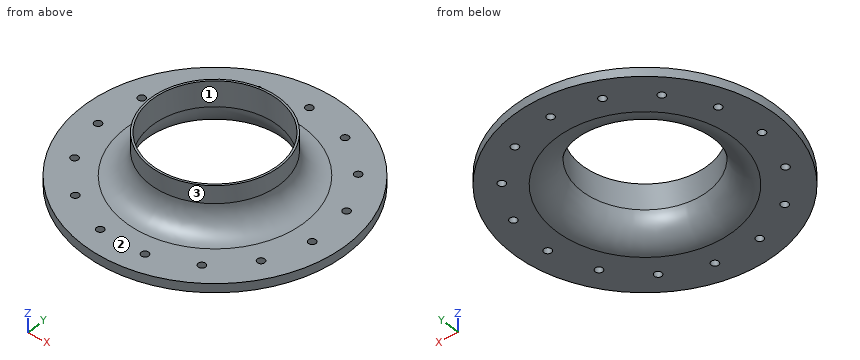
from build123d import *

# Parameters (mm, degrees)
ESQUISSE2_R             = 1.5
ENL_V_MAT_EXTRU_1_DEPTH = 78.521900132


with BuildPart() as part:
    # Esquisse1 → Base-Révolution (revolve)
    with BuildSketch(Plane(origin=(0, 0, 0), x_dir=(0, 0, -1), z_dir=(1, 0, 0)), mode=Mode.PRIVATE) as base_r_volution_sk:
        with BuildLine():
            Line((20.85, 46.5), (20.85, 53.45))
            Line((20.85, 53.45), (17.2, 53.45))
            Line((17.2, 53.45), (17.2, 36.3))
            ThreePointArc((17.2, 36.3), (14.271067812, 29.228932188), (7.2, 26.3))
            Line((7.2, 26.3), (0, 26.3))
            Line((0, 26.3), (0, 25.5))
            Line((0, 25.5), (1.5, 25.5))
            Line((1.5, 25.5), (10.35, 25.5))
            ThreePointArc((10.35, 25.5), (17.774621202, 28.575378798), (20.85, 36))
            Line((20.85, 36), (20.85, 46.5))
        make_face()
    revolve(base_r_volution_sk.sketch.rotate(Axis((0, 0, 0), (0, 0, -1)), 90), axis=Axis((0, 0, 0), (0, 0, -1)))

    # Esquisse2 → Enlèv. mat.-Extru.1 (cut, through all)
    with BuildSketch(Plane.XY.offset(-17.2)):
        with Locations((0, 44.5)):
            Circle(ESQUISSE2_R)
        with Locations((18.099780617, 40.652772865)):
            Circle(ESQUISSE2_R)
        with Locations((33.069944734, 29.776311983)):
            Circle(ESQUISSE2_R)
        with Locations((42.322014975, 13.75125625)):
            Circle(ESQUISSE2_R)
        with Locations((44.256224344, -4.651516615)):
            Circle(ESQUISSE2_R)
        with Locations((38.538130468, -22.25)):
            Circle(ESQUISSE2_R)
        with Locations((26.156443727, -36.00125625)):
            Circle(ESQUISSE2_R)
        with Locations((9.252070241, -43.527568233)):
            Circle(ESQUISSE2_R)
        with Locations((-9.252070241, -43.527568233)):
            Circle(ESQUISSE2_R)
        with Locations((-26.156443727, -36.00125625)):
            Circle(ESQUISSE2_R)
        with Locations((-38.538130468, -22.25)):
            Circle(ESQUISSE2_R)
        with Locations((-44.256224344, -4.651516615)):
            Circle(ESQUISSE2_R)
        with Locations((-42.322014975, 13.75125625)):
            Circle(ESQUISSE2_R)
        with Locations((-33.069944734, 29.776311983)):
            Circle(ESQUISSE2_R)
        with Locations((-18.099780617, 40.652772865)):
            Circle(ESQUISSE2_R)
    extrude(amount=-ENL_V_MAT_EXTRU_1_DEPTH, mode=Mode.SUBTRACT)


solid = part.part
Source: CAD feature listing. Evaluate the final solid. Frame: model axes, mm. Face numbers are marked on the shaded views. Round coordinates to 2 decimals unless told otherwise and drop trailing zeros. Loops run counter-clockwise (first coordinate to the right, second up) from the corner with the lowest first, then second, coordinate; pieces in that order, holes last. Notation, with made-up numbers: M 54,73.25 L 65,73.25 A16 ccw 65,84.25 Z; hole C 6.25,-26 d1. An arc over 180 degrees is marked long. Return JSON: item names as keys, results as strings. Group by question number.
1. Section query D-D on y = 44.5. Output: boundary loops of the cut face in (x, z), and give its area (3 significant figures).
2. Pin query (flat end, axial travel): pin 1 (12 mm diameter, centred on x = -18, z = -9, fed in from -Y); pin 2 (4 mm diameter, centred on x = 1.5, z = -3.5, fed in from -Y); pin 3 (5 mm diameter, centred on x = 2.5, z = -8, fed in from -Y). Return the tip coordinate at first contact, or that it passes through.
3. Section query C-C on z = -1.5. Output: boundary loops of the cut face in (x, y), and give its area (3 significant figures).
4. Section query A-A on x = 0. Output: boundary loops of the cut face in (y, z).
5. Material intervals for line 1 along Y through (x, z) = (-6.5, -4.5); line 2 along X through (y, z) = (15, -18.75); line 3 along X through (y, z) = (-12, -18.75), sorted ascending. Write a range as from..to.
6. Mould query, pull axis X, two halves, no side actions, for the marked faces 1, 2 and 3. Classes: released by +X, released by -X, zero draft, split by the parting line, or undercut.
7. Section query B-B on y = 0. Output: boundary loops of the cut face in (x, z), and give its area (3 significant figures).
Checks:
{
 "1": {"outline": "M -29.61,-20.85 L -1.5,-20.85 L -1.5,-17.2 L -29.61,-17.2 Z; M 1.5,-20.85 L 29.61,-20.85 L 29.61,-17.2 L 1.5,-17.2 Z", "area": "205 mm²"},
 "2": {"pin 1": "stops at y = -25.01", "pin 2": "stops at y = -26.3", "pin 3": "stops at y = -26.77"},
 "3": {"outline": "C 0,0 d52.6; hole C 0,0 d51", "area": "130 mm²"},
 "4": {"outline": "M -53.45,-20.85 L -36,-20.85 A10.5 ccw -25.5,-10.35 L -25.5,0 L -26.3,0 L -26.3,-7.2 A10 cw -36.3,-17.2 L -53.45,-17.2 Z; M 25.5,-10.35 A10.5 ccw 36,-20.85 L 43,-20.85 L 43,-17.2 L 36.3,-17.2 A10 cw 26.3,-7.2 L 26.3,0 L 25.5,0 Z; M 46,-20.85 L 53.45,-20.85 L 53.45,-17.2 L 46,-17.2 Z"},
 "5": {"line 1": "y = -25.48..-24.66, 24.66..25.48", "line 2": "x = -51.3..-43.15, -41.49..-25.63, 25.63..41.49, 43.15..51.3", "line 3": "x = -52.09..-27.17, 27.17..52.09"},
 "6": {"face 1": "undercut", "face 2": "zero draft", "face 3": "split by the parting line"},
 "7": {"outline": "M -53.45,-20.85 L -36,-20.85 A10.5 ccw -25.5,-10.35 L -25.5,0 L -26.3,0 L -26.3,-7.2 A10 cw -36.3,-17.2 L -53.45,-17.2 Z; M 25.5,-10.35 A10.5 ccw 36,-20.85 L 53.45,-20.85 L 53.45,-17.2 L 36.3,-17.2 A10 cw 26.3,-7.2 L 26.3,0 L 25.5,0 Z", "area": "227 mm²"}
}
